```python
from build123d import *

# Parameters (mm, degrees)
SKETCH1_R           = 3
BOSS_EXTRUDE1_DEPTH = 3.7
SKETCH1_3_R         = 1.6
BOSS_EXTRUDE2_DEPTH = 1
SKETCH5_R           = 1.5
BOSS_EXTRUDE3_DEPTH = 1
SKETCH6_R           = 2
BOSS_EXTRUDE4_DEPTH = 1
SKETCH8_R           = 1.5
BOSS_EXTRUDE5_DEPTH = 2
SKETCH10_R          = 1.8
BOSS_EXTRUDE6_DEPTH = 1
SKETCH12_R          = 1.65
CUT_EXTRUDE1_DEPTH  = 2


with BuildPart() as part:
    # Sketch1 → Boss-Extrude1 (new body)
    with BuildSketch(Plane(origin=(0, 0, 0), x_dir=(1, 0, 0), z_dir=(0, 1, 0))):
        with Locations((-0.522013312, 0.511138034)):
            Circle(SKETCH1_R)
    extrude(amount=BOSS_EXTRUDE1_DEPTH)

    # Sketch1<3> → Boss-Extrude2 (add)
    with BuildSketch(Plane(origin=(0, 0, 0), x_dir=(1, 0, 0), z_dir=(0, 1, 0))):
        with Locations((-0.522013312, 0.511138034)):
            Circle(SKETCH1_3_R)
    extrude(amount=BOSS_EXTRUDE2_DEPTH)

    # Sketch5 → Boss-Extrude3 (add)
    with BuildSketch(Plane.XZ):
        with Locations((-0.522013312, -0.511138034)):
            Circle(SKETCH5_R)
    extrude(amount=BOSS_EXTRUDE3_DEPTH)

    # Sketch6 → Boss-Extrude4 (add)
    with BuildSketch(Plane.XZ.offset(1)):
        with Locations((-0.522013312, -0.511138034)):
            Circle(SKETCH6_R)
    extrude(amount=BOSS_EXTRUDE4_DEPTH)

    # Sketch8 → Boss-Extrude5 (add)
    with BuildSketch(Plane(origin=(0, -2, 0), x_dir=(-1, 0, 0), z_dir=(0, -1, 0))):
        with Locations((0.522013312, 0.511138034)):
            Circle(SKETCH8_R)
    extrude(amount=BOSS_EXTRUDE5_DEPTH)

    # Sketch10 → Boss-Extrude6 (add)
    with BuildSketch(Plane.XZ.offset(4)):
        with Locations((-0.522013312, -0.511138034)):
            Circle(SKETCH10_R)
    extrude(amount=-BOSS_EXTRUDE6_DEPTH)

    # Sketch12 → Cut-Extrude1 (cut)
    with BuildSketch(Plane(origin=(0, 3.7, 0), x_dir=(1, 0, 0), z_dir=(0, 1, 0))):
        with Locations((-0.522013312, 0.511138034)):
            Circle(SKETCH12_R)
    extrude(amount=-CUT_EXTRUDE1_DEPTH, mode=Mode.SUBTRACT)


solid = part.part
```
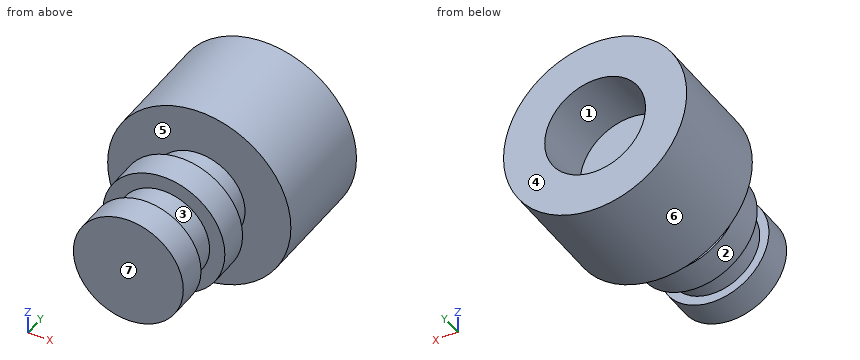
The model under review builds one solid part; all positions refer to its coordinate system, in mm. Face numbers are marked on the shaded views. A direction names the side the tool comes from. Round coordinates to 2 decimals unless told otherwise and drop trailing zeros. Order: outer loops, then holes, each group sorted by start corner. A loop starts at its lowest first (then second) coordinate and runs counter-clockwise, first axis right, second up. Notation, with made-up numbers: (36.5, 5.25) -> (94.5, 5.25) arc R25 cw to (94.5, 41.25) -> close; hole circle Ø7 at (79, 72.25). An arc over 180 degrees is marked (long way). Use a Markdown table: item, result.
Q1. For line 1 (Y direction, x = 0.25, z = 0.9); line 2 (Y direction, x = -0.7, z = -2.45); line 3 (Z direction, x = -0.6, y = 2), list the stretches that pass through material, from the lowest coordinate up.
Values:
| item | result |
|---|---|
| line 1 | y = -4 to -3, -2 to -1, 0 to 1.7 |
| line 2 | y = -2 to -1, 0 to 3.7 |
| line 3 | z = -3.51 to -2.16, 1.14 to 2.49 |
Q2. Clearance check with flat-ended pins moving along their axes: P1, Ø1.2, axis at x = -1, z = -1, coming from the +Y side; P2, Ø2.5, axis at x = -1, z = -1, coming from the +Y side. State where each tip first meets the part, or that it passes through.
Values:
| item | result |
|---|---|
| P1 | stops at y = 1.7 |
| P2 | stops at y = 3.7 |
Q3. We need section A-A on x = 0.7. Write out the cut boundary in (y, z).
Values:
| item | result |
|---|---|
| outline | (-4, -1.83) -> (-3, -1.83) -> (-3, -1.38) -> (-2, -1.38) -> (-2, -2.09) -> (-1, -2.09) -> (-1, -1.38) -> (0, -1.38) -> (0, -3.25) -> (3.7, -3.25) -> (3.7, -1.62) -> (1.7, -1.62) -> (1.7, 0.6) -> (3.7, 0.6) -> (3.7, 2.23) -> (0, 2.23) -> (0, 0.36) -> (-1, 0.36) -> (-1, 1.07) -> (-2, 1.07) -> (-2, 0.36) -> (-3, 0.36) -> (-3, 0.81) -> (-4, 0.81) -> close |
Q4. Mouldability with a two-part tool opening along Y and no side actions: class the marked faces 4, 5, 6 and 7 as +Y half, -Y half, draft (parallel to the pull), parting line (faces both ways), or undercut.
Values:
| item | result |
|---|---|
| face 4 | +Y half |
| face 5 | undercut |
| face 6 | draft |
| face 7 | -Y half |
Q5. We need section C-C on y = 2. Write out the cut boundary in (x, z).
Values:
| item | result |
|---|---|
| outline | circle Ø6 at (-0.52, -0.51); hole circle Ø3.3 at (-0.52, -0.51) |
Q6. We need section D-D on y = -0.75. Write out the cut boundary in (x, z).
Values:
| item | result |
|---|---|
| outline | circle Ø3 at (-0.52, -0.51) |
Q7. Tool access review of the marked faces 1, 2 and 3: name each direction out of +Z, -Z, +X, -X, +Y, -Y from which nothing blocks a thin tool from reaching the whole face with its end or side.
Values:
| item | result |
|---|---|
| face 1 | +Y |
| face 2 | -Y |
| face 3 | none |
Q8. We need section B-B on z = -0.25. Write out the cut boundary in (x, y).
Values:
| item | result |
|---|---|
| outline | (-3.51, 0) -> (-2, 0) -> (-2, -1) -> (-2.5, -1) -> (-2.5, -2) -> (-2, -2) -> (-2, -3) -> (-2.3, -3) -> (-2.3, -4) -> (1.26, -4) -> (1.26, -3) -> (0.96, -3) -> (0.96, -2) -> (1.46, -2) -> (1.46, -1) -> (0.96, -1) -> (0.96, 0) -> (2.47, 0) -> (2.47, 3.7) -> (1.11, 3.7) -> (1.11, 1.7) -> (-2.15, 1.7) -> (-2.15, 3.7) -> (-3.51, 3.7) -> close |
